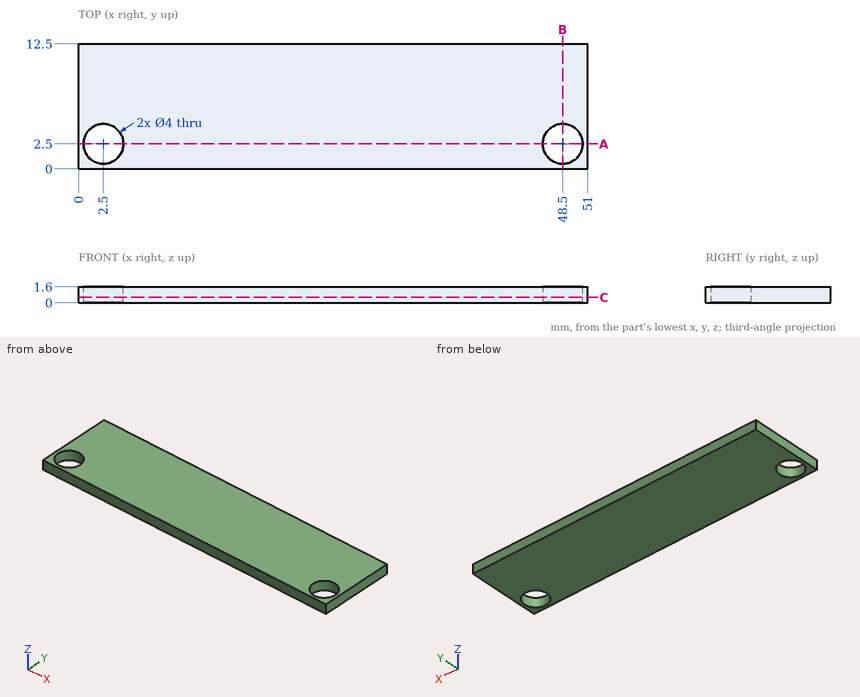
Here's the drawing with two shaded views (mm, measured from the low corner). I have some questions. Give positions to 0.01 mm unless a question says otherwise; leave off trailing zeros. Order: outer loops, then holes, each group sorted by start corner. A loop starts at its lowest first (then second) coordinate and runs counter-clockwise, first axis right, second up. Notation, with made-up numbers: M 80.25,46.25 L 95.25,46.25 A15 cw 95.25,67.25 Z; hole C -11.75,-2.75 d8. An arc over 180 degrees is marked long. One line per question, with ' | ' between items.
Item 1: Suppose I cut it at C-C, the plane z = 0.55. Write out the boundary of the cut face in (x, y).
Answer block:
outline: M 0,0 L 51,0 L 51,12.5 L 0,12.5 Z; hole C 2.5,2.5 d4; hole C 48.5,2.5 d4
Item 2: Suppose I cut it at B-B, the plane x = 48.5. Write out the boundary of the cut face in (y, z), then the cut area to 3 significant figures.
Answer block:
outline: M 0,0 L 0.5,0 L 0.5,1.6 L 0,1.6 Z; M 4.5,0 L 12.5,0 L 12.5,1.6 L 4.5,1.6 Z | area: 13.6 mm2
Item 3: Please list where these lines run through material, in increasing order: L1, parallel to X at y = 2.5, z = 1.05; L2, parallel to Y at x = 48.5, z = 1.15; L3, parallel to X at y = 1.5, z = 0.9.
Answer block:
L1: x = 0 to 0.5, 4.5 to 46.5, 50.5 to 51 | L2: y = 0 to 0.5, 4.5 to 12.5 | L3: x = 0 to 0.77, 4.23 to 46.77, 50.23 to 51
Item 4: Suppose I cut it at A-A, the plane y = 2.5. Write out the boundary of the cut face in (x, z), then the cut area to 3 significant figures.
Answer block:
outline: M 0,0 L 0.5,0 L 0.5,1.6 L 0,1.6 Z; M 4.5,0 L 46.5,0 L 46.5,1.6 L 4.5,1.6 Z; M 50.5,0 L 51,0 L 51,1.6 L 50.5,1.6 Z | area: 68.8 mm2
